Autodesk Inventor part; units mm, degrees
ref_plane "YZ Plane" through (0, 0, 0) normal (1, 0, 0) x (0, 1, 0)
ref_plane "XZ Plane" through (0, 0, 0) normal (0, 1, 0) x (-1, 0, 0)
ref_plane "XY Plane" through (0, 0, 0) normal (0, 0, 1) x (1, 0, 0)
sketch "スケッチ1" plane through (0, 0, 0) normal (0, 1, 0) x (-1, 0, 0)
  line L0 (-75, -90) -> (75, -90)
  line L1 (75, -90) -> (75, 90)
  line L2 (75, 90) -> (-75, 90)
  line L3 (-75, 90) -> (-75, -90)
  line L4 (-75, -90) -> (75, 90) construction
  line L5 (75, -90) -> (-75, 90) construction
  point P0 (0, 0)
  dimension "d0" = 150
  dimension "d1" = 180
extrude "押し出し1" add sketch "スケッチ1" along normal blind 4
sketch "スケッチ2" plane through (0, 4, 0) normal (0, 1, 0) x (1, 0, 0)
  line L0 (-75, -90) -> (75, -90)
  line L1 (-62.6, -90) -> (62.6, -90)
  line L2 (62.6, -90) -> (62.6, 10)
  line L3 (62.6, 10) -> (-62.6, 10)
  line L4 (-62.6, 10) -> (-62.6, -90)
  point P0 (0, 0)
  dimension "d4" = 125.2
  dimension "d5" = 100
  dimension "d6" = 62.6
extrude "押し出し2" cut sketch "スケッチ2" against normal blind 4
sketch "スケッチ3" plane through (0, 0, 0) normal (0, -1, 0) x (1, 0, 0)
  line L0 (62.6, 90) -> (75, 90)
  line L1 (72, 90) -> (65.8, 90)
  line L2 (65.8, 90) -> (65.8, -90)
  line L3 (65.8, -90) -> (72, -90)
  line L4 (72, -90) -> (72, 90)
  line L5 (75, 90) -> (75, -90)
  line L6 (0, 0) -> (0, 35.088)
  line L7 (-62.6, 90) -> (-75, 90)
  line L8 (-72, 90) -> (-65.8, 90)
  line L9 (-65.8, 90) -> (-65.8, -90)
  line L10 (-65.8, -90) -> (-72, -90)
  line L11 (-72, -90) -> (-72, 90)
  line L12 (-75, 90) -> (-75, -90)
  dimension "d9" = 6.2
  dimension "d10" = 180
  dimension "d11" = 3
extrude "押し出し3" cut sketch "スケッチ3" against normal blind 2
sketch "スケッチ4" plane through (0, 4, 0) normal (0, 1, 0) x (1, 0, 0)
  line L0 (62.6, 10) -> (-62.6, 10)
  line L1 (-4.5, 10) -> (4.5, 10)
  line L2 (4.5, 10) -> (4.5, -90)
  line L3 (4.5, -90) -> (-4.5, -90)
  line L4 (-4.5, -90) -> (-4.5, 10)
  point P0 (0, 0)
  dimension "d14" = 9
  dimension "d15" = 100
  dimension "d16" = 4.5
extrude "押し出し4" add sketch "スケッチ4" against normal blind 4
sketch "スケッチ5" plane through (0, 4, 0) normal (0, 1, 0) x (1, 0, 0)
  circle A0 centre (0, -5.589) radius 121.5
  line L0 (75, 90) -> (72, 90)
  line L1 (-75, 90) -> (-75, -90)
  line L2 (-75, 90) -> (75, 90)
  point P0 (0, 0)
  dimension "d19" = 243
extrude "押し出し5" add sketch "スケッチ5" against normal blind 4 contours L0 L2 A0 picked at (-21.9725, 92.7838)
sketch "スケッチ6" plane through (0, 4, 0) normal (0, 1, 0) x (1, 0, 0)
  arc A0 (75, 90) -> (-75, 90) centre (0, -5.589) ccw
  line L0 (75, 90) -> (-75, 90) construction
  line L1 (0, 90) -> (0, 115.911) construction
  point P0 (0, 0)
  point P1 (0, 102)
  point P2 (30, 102)
  point P3 (-30, 102)
  dimension "d22" = 12
  dimension "d23" = 30
hole "穴1" at (75, 4, -90) at (0, 4, -102) at (30, 4, -102) at (-30, 4, -102) direction (0, -1, 0) diameter 3.2 end through all
sketch "スケッチ7" plane through (0, 4, 0) normal (0, 1, 0) x (1, 0, 0)
  line L0 (-62.6, 10) -> (-4.5, 10)
  line L1 (-62.6, 14) -> (62.6, 14)
  line L2 (62.6, 14) -> (62.6, 89)
  line L3 (-62.6, 89) -> (-62.6, 14)
  arc A0 (62.6, 89) -> (-62.6, 89) centre (0, -137.2653) ccw
  line L4 (-59.6, 14) -> (62.6, 86)
  line L5 (-62.6, 17) -> (60.547, 89.558)
  line L6 (0, 14) -> (0, 41.0158)
  line L7 (59.6, 14) -> (-62.6, 86)
  line L8 (62.6, 17) -> (-60.547, 89.558)
  point P0 (0, 0)
  point P1 (0, 97.5)
  point P2 (0, 53.8838)
  point P3 (-4.0458, 51.5)
  point P4 (0, 49.1162)
  point P5 (4.0458, 51.5)
  dimension "d32" = 4
  dimension "d33" = 125.2
  dimension "d34" = 75
  dimension "d36" = 3
  dimension "d37" = 3
  dimension "d38" = 3
extrude "押し出し6" cut sketch "スケッチ7" against normal blind 4 contours L4 L7 L1 | L3 L7 L5 | L4 L2 L8 | L8 A0 L5
sketch "スケッチ8" plane through (0, 4, 0) normal (0, 1, 0) x (1, 0, 0)
  line L0 (-62.6, 10) -> (-4.5, 10)
  point P0 (0, 0)
  point P1 (0, 0)
  point P2 (0, -40)
  point P3 (0, -80)
  dimension "d41" = 10
  dimension "d42" = 50
  dimension "d43" = 90
hole "穴2" at (0, 4, 0) at (0, 4, 40) at (0, 4, 80) direction (0, -1, 0) diameter 3.2 end through all
fillet "フィレット1" radius 4 2 edges at (0, 2, -49.1162) (0, 2, -53.8838)
properties part number "お盆4" material "アルミニウム 2014-T6"
Could you check a few things on this model? Use its own coordinates, in mm. A direction names the side the tool comes from. Coordinates: 2 decimals unless noted, no trailing zeros. Write each loop counter-clockwise with the first axis right and the second up, starting at its lowest first coordinate (ties: lowest second). Pieces come first, ordered by that corner, then holes. Notation, with made-up numbers: (23.5, -27) - (43.5, -27) arc R20 ccw to (43.5, -18) - close; hole circle Ø11 at (-34, -25.5). An arc over 180 degrees is marked (long way). Write item = value, one per line.
1) Suppose I cut it at D-D on z = -26. Please give me the cut outline in (x, y) (3 decimals).
Result set:
outline = (-75, 0) - (-72, 0) - (-72, 2) - (-65.8, 2) - (-65.8, 0) - (-62.6, 0) - (-62.6, 4) - (-75, 4) - close; (-47.325, 0) - (-39.233, 0) - (-39.233, 4) - (-47.325, 4) - close; (39.233, 0) - (47.325, 0) - (47.325, 4) - (39.233, 4) - close; (62.6, 0) - (65.8, 0) - (65.8, 2) - (72, 2) - (72, 0) - (75, 0) - (75, 4) - (62.6, 4) - close
2) For faces 1 (the flat face through (69, 2, 1)), 2 (the flat face through (34, 2, -10)), 3 (the flat face through (-32.9, 2, -68.5)), which set-ups out of +Z, -Z, +X, -X, +Y, -Y let a thin tool reach every point of the face, with its end or its side?
Result set:
face_1 = +Z, -Y
face_2 = +Z, +Y, -Y
face_3 = +Y, -Y
3) Suppose I cut it at C-C on x = 14. Please give me the cut outline in (y, z).
Result set:
outline = (0, -115.1) - (4, -115.1) - (4, -97.08) - (0, -97.08) - close; (0, -62.13) - (4, -62.13) - (4, -57.36) - (0, -57.36) - close; (0, -45.64) - (4, -45.64) - (4, -40.87) - (0, -40.87) - close; (0, -14) - (4, -14) - (4, -10) - (0, -10) - close
4) Please list where these lines run through material, in increasing order: line 1 (X direction, y = 0.45, z = 42); line 2 (X direction, y = 0.9, z = 80); line 3 (X direction, y = 3.8, z = 48). Write a range as [from, to].
Result set:
line_1 = [-75, -72], [-65.8, -62.6], [-4.5, 4.5], [62.6, 65.8], [72, 75]
line_2 = [-75, -72], [-65.8, -62.6], [-4.5, -1.6], [1.6, 4.5], [62.6, 65.8], [72, 75]
line_3 = [-75, -62.6], [-4.5, 4.5], [62.6, 75]
5) Suppose I cut it at B-B on y = 3.1. State how many separate pieces and enclosed holes the cut face has, plus the area to 3 significant figures.
Result set:
separate_pieces = 1
enclosed_holes = 10
area = 9,050 mm2
6) Suppose I cut it at A-A on z = 56. Please give me the cut outline in (x, y), plus the area to 3 significant figures.
Result set:
outline = (-75, 0) - (-72, 0) - (-72, 2) - (-65.8, 2) - (-65.8, 0) - (-62.6, 0) - (-62.6, 4) - (-75, 4) - close; (-4.5, 0) - (4.5, 0) - (4.5, 4) - (-4.5, 4) - close; (62.6, 0) - (65.8, 0) - (65.8, 2) - (72, 2) - (72, 0) - (75, 0) - (75, 4) - (62.6, 4) - close
area = 110 mm2
7) We'd pull the mould along X, two halves only. Please class faces 4 (the flat face through (75, 2, 2)), 5 (the flat face through (-62.6, 2, -52)), 6 (the flat face through (68.7, 2.4, 90)): +X half, -X half, draft (parallel to the pull), parting line (faces both ways), or undercut.
Result set:
face_4 = +X half
face_5 = undercut
face_6 = draft
8) Will these pins go through, and if not, where does the flat tip stop? pin 1 Ø1.6 at (x, y) = (68, 1) entering from +Z; pin 2 Ø1.9 at (x, z) = (30, -102) entering from -Y; pin 3 Ø5 at (x, z) = (69, -34) entering from -Y.
Result set:
pin_1 = -90
pin_2 = through
pin_3 = 2
